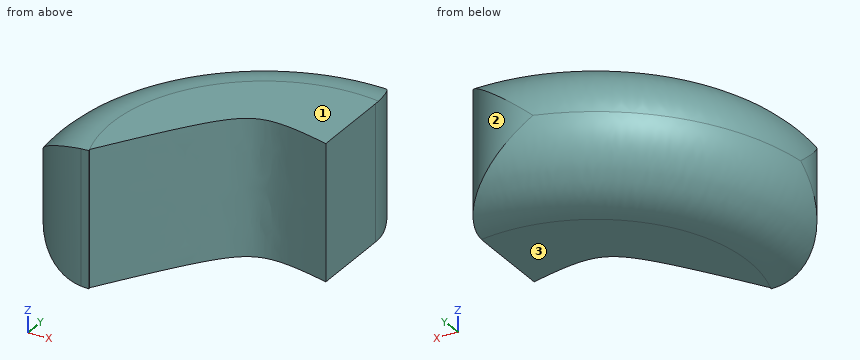
from build123d import *

# Parameters (mm, degrees)
BOSS_EXTRUDE1_DEPTH = 5.08
FILLET1_R           = 2.54
CUT_EXTRUDE1_DEPTH  = 5.08


with BuildPart() as part:
    # Sketch2 → Boss-Extrude1 (new body)
    with BuildSketch(Plane.XY):
        with BuildLine():
            Line((0, 0), (-8.89, 0))
            ThreePointArc((-8.89, 0), (-7.067912046, 7.37504804), (0, 10.16))
            Line((0, 10.16), (0, 0))
        make_face()
    extrude(amount=BOSS_EXTRUDE1_DEPTH)

    # Fillet1
    fillet1_edges = [part.edges().sort_by_distance(p)[0] for p in [
        (-7.067912046, 7.37504804, 0),
        (-8.89, 0, 2.54),
        (0, 10.16, 2.54),
        (-7.067912046, 7.37504804, 5.08),
    ]]
    fillet(fillet1_edges, radius=FILLET1_R - 0.0001)  # a hair under: the kernel refuses the full size

    # Sketch4 → Cut-Extrude1 (cut)
    with BuildSketch(Plane.XY):
        with BuildLine():
            Line((0, 4.342456755), (0, 0))
            Line((0, 0), (-6.244672338, 0))
            Line((-6.244672338, 0), (-6.270779923, 0.075057389))
            add(Edge.make_bspline(
                [(-6.270779923, 0.075057389), (-3.105835382, 5.113383938), (0, 4.342456755)],
                knots=[0, 0, 0, 1, 1, 1], degree=2, weights=[1, 3, 1]))
        make_face()
    extrude(amount=CUT_EXTRUDE1_DEPTH, mode=Mode.SUBTRACT)


solid = part.part
Build history of the part. All positions in model axes, mm. Face numbers are marked on the shaded views. Coordinates: 2 decimals unless noted, no trailing zeros. One line per question, with ' | ' between items. Start each with the question number.
Q1. Probe L1, parallel to Z at x = -4.75, y = 6.5; L2, parallel to Y at x = -6, z = 1.85; L3, parallel to Y at x = -3, z = 1.7. List the from-to ranges inside material, lowest first. Write a range as from..to.
Q2. Flat gauge pin, fed straight in: pin 1 Ø1.5 at (y, z) = (6, 4) entering from -X. Where does the tip first touch, or does it go through?
Q3. Two-plate mould, pull along Z, no slides. Class the marked faces 1, 2 and 3: +Z half, -Z half, draft (parallel to the pull), parting line (faces both ways), or undercut.
Check values:
1) L1: z = 0.02..5.06 | L2: y = 0.5..8.27 | L3: y = 4.46..9.77
2) pin 1: stops at x = -8.12
3) face 1: +Z half | face 2: draft | face 3: -Z half
